Build history of the part. All positions in model axes, mm. A direction names the side the tool comes from. Round coordinates to 2 decimals unless told otherwise and drop trailing zeros. Order: outer loops, then holes, each group sorted by start corner. A loop starts at its lowest first (then second) coordinate and runs counter-clockwise, first axis right, second up. Notation, with made-up numbers: (83.5, -6) - (142.5, -6) arc R29 ccw to (142.5, 17) - close; hole circle Ø8 at (63, -6). An arc over 180 degrees is marked (long way). One line per question, with ' | ' between items. Start each with the question number.
from build123d import *

# Parameters (mm, degrees)
SKETCH1_W                          = 31.9532
SKETCH1_H                          = 31.75
EXTRUDE1_DEPTH                     = 9.525
SKETCH2_R                          = 6.35
EXTRUDE2_DEPTH                     = 6.35
CHAMFER1_SIZE                      = 3.175
F_3_4_10_ACME_2C_RH_TAPPED_HOLE1_D = 19.05
CHAMFER2_SIZE                      = 2.3622


with BuildPart() as part:
    # Sketch1 → Extrude1 (new body, symmetric)
    with BuildSketch(Plane.XY):
        Rectangle(SKETCH1_W, SKETCH1_H)
    extrude(amount=EXTRUDE1_DEPTH, both=True)

    # Sketch2 → Extrude2 (add)
    with BuildSketch(Plane.ZY.offset(15.9766)):
        with Locations(Location((0, 0, 0), (0, 0, 90))):  # turned: the seam where the file's is
            Circle(SKETCH2_R)
    extrude2 = extrude(amount=EXTRUDE2_DEPTH)

    # Mirror1: Extrude2 across plane
    add(extrude2.mirror(Plane(origin=(0, 0, 0), x_dir=(0, 0, 1), z_dir=(1, 0, 0))))

    # Chamfer1
    chamfer1_edges = [part.edges().sort_by_distance(p)[0] for p in [
        (0, 15.875, -9.525),
        (0, -15.875, -9.525),
    ]]
    chamfer(chamfer1_edges, length=CHAMFER1_SIZE)

    # 3/4-10-ACME-2C-RH Tapped Hole1 (through all)
    with Locations(Plane.XY.offset(9.525)):
        with Locations((0, 0)):
            Hole(F_3_4_10_ACME_2C_RH_TAPPED_HOLE1_D / 2)

    # Chamfer2
    chamfer2_edges = [part.edges().sort_by_distance(p)[0] for p in [
        (15.9766, 0, 9.525),
        (-15.9766, 0, 9.525),
    ]]
    chamfer(chamfer2_edges, length=CHAMFER2_SIZE)


solid = part.part
Item 1: Slice it at A-A (z = 0). Write the cut outline in (x, y) (3 decimals).
Item 2: 3-axis set-ups, long thin cutter, end or side, ignore diameter. For faces 1 (the face through (-19.11, -5.04, 3.86)), 2 (the face through (19.11, -5.04, 3.86)), 3 (the face through (-0.224, -14.265, -7.96)): which of +Z, -Z, +X, -X, +Y, -Y reach the whole face in a straight line?
Item 3: Slice it at B-B (x = 0). Write the cut outline in (y, z) (3 decimals).
Item 4: Wall check: line 1 along Y through (x, z) = (0, 2) (3 decimals); line 2 along X through (y, z) = (-12.5, -1); line 3 along X through (y, z) = (5, 5). Give the ranges that are in metal, low to high. Write a range as [from, to].
Item 5: Slice it at C-C (y = 0). Write the cut outline in (x, z) (3 decimals), plus the area to 3 significant figures.
Item 6: Pull direction X, two halves, no side cores. Call faces 4 (the face through (14.81, -0.22, 8.33)), 5 (the face through (-15.977, 0, -7)), 6 (the face through (0, 15.875, 2)), 7 (the face through (7.559, -5.796, -0.133)): released by +X, released by -X, zero draft, split by the parting line, or undercut.
Item 7: Pin check, flat tips, straight feed: pin 1 (5 mm diameter, centred on y = 6.5, z = 2.5, fed in from +X); pin 2 (2 mm diameter, centred on y = -11, z = 1.5, fed in from -X); pin 3 (3 mm diameter, centred on x = 4.5, y = 5, fed in from +Z). Stop position of each tip, or through.
Item 8: Slice it at D-D (y = 7). Write the cut outline in (x, z) (3 decimals).
A:
1) outline: (-22.327, -6.35) - (-15.977, -6.35) - (-15.977, -15.875) - (15.977, -15.875) - (15.977, -6.35) - (22.327, -6.35) - (22.327, 6.35) - (15.977, 6.35) - (15.977, 15.875) - (-15.977, 15.875) - (-15.977, 6.35) - (-22.327, 6.35) - close; hole circle Ø19.05 at (0, 0)
2) face 1: -X | face 2: +X | face 3: -Z, +X, -X, -Y
3) outline: (-15.875, -6.35) - (-12.7, -9.525) - (-9.525, -9.525) - (-9.525, 9.525) - (-15.875, 9.525) - close; (9.525, -9.525) - (12.7, -9.525) - (15.875, -6.35) - (15.875, 9.525) - (9.525, 9.525) - close
4) line 1: [-15.875, -9.525], [9.525, 15.875] | line 2: [-15.98, 15.98] | line 3: [-15.98, -8.11], [8.11, 15.98]
5) outline: (-22.327, -6.35) - (-15.977, -6.35) - (-15.977, -9.525) - (-9.525, -9.525) - (-9.525, 9.525) - (-13.614, 9.525) - (-15.977, 7.163) - (-15.977, 6.35) - (-22.327, 6.35) - close; (9.525, -9.525) - (15.977, -9.525) - (15.977, -6.35) - (22.327, -6.35) - (22.327, 6.35) - (15.977, 6.35) - (15.977, 7.163) - (13.614, 9.525) - (9.525, 9.525) - close | area: 402 mm^2
6) face 4: released by +X | face 5: released by -X | face 6: zero draft | face 7: undercut
7) pin 1: x = 22.33 | pin 2: x = -15.98 | pin 3: through
8) outline: (-15.977, -9.525) - (-6.46, -9.525) - (-6.46, 9.525) - (-13.614, 9.525) - (-15.977, 7.163) - close; (6.46, -9.525) - (15.977, -9.525) - (15.977, 7.163) - (13.614, 9.525) - (6.46, 9.525) - close
